Read the model definition and answer for the solid it produces. Units are mm, in the model's axes. A direction names the side the tool comes from. Coordinates: 2 decimals unless noted, no trailing zeros. Order: outer loops, then holes, each group sorted by start corner. A loop starts at its lowest first (then second) coordinate and runs counter-clockwise, first axis right, second up. Notation, with made-up numbers: (21, 56) -> (64, 56) arc R24 ccw to (64, 71) -> close; hole circle Ø3 at (72.25, 21). An arc over 180 degrees is marked (long way). Use CSV: the item, a comma, the result in double quotes.
```python
from build123d import *

# Parameters (mm, degrees)
SKETCH1_W           = 94
SKETCH1_H           = 48
BOSS_EXTRUDE1_DEPTH = 10
CUT_EXTRUDE1_DEPTH  = 6
SKETCH3_W           = 2.75
SKETCH3_H           = 8.5
CUT_EXTRUDE2_DEPTH  = 10
SKETCH4_R           = 2.5
BOSS_EXTRUDE2_DEPTH = 1.7
SKETCH5_R           = 2.5
BOSS_EXTRUDE3_DEPTH = 1.7
SKETCH6_R           = 2.5
CUT_EXTRUDE3_DEPTH  = 10
SKETCH11_R          = 3.2
CUT_EXTRUDE4_DEPTH  = 1
CUT_EXTRUDE5_START  = -10
SKETCH12_R          = 2.5
CUT_EXTRUDE5_DEPTH  = 10
CUT_EXTRUDE6_START  = -1
SKETCH13_R          = 3.2
CUT_EXTRUDE6_DEPTH  = 1
SKETCH15_W          = 20.2
SKETCH15_H          = 6.1
CUT_EXTRUDE7_DEPTH  = 2.1
CUT_EXTRUDE9_DEPTH  = 12
SKETCH19_W          = 11.1
SKETCH19_H          = 4.1
CUT_EXTRUDE10_DEPTH = 7.9
CUT_EXTRUDE11_DEPTH = 4.1


with BuildPart() as part:
    # Sketch1 → Boss-Extrude1 (new body)
    with BuildSketch(Plane(origin=(0, 0, 0), x_dir=(1, 0, 0), z_dir=(0, 1, 0))):
        Rectangle(SKETCH1_W, SKETCH1_H)
    extrude(amount=BOSS_EXTRUDE1_DEPTH)

    # Sketch2 → Cut-Extrude1 (cut)
    with BuildSketch(Plane(origin=(0, 10, 0), x_dir=(1, 0, 0), z_dir=(0, 1, 0))):
        Polygon((-21.568604419, -3.5), (-5.068604419, -3.5), (-5.068604419, -20), (-21.568604419, -20), (-21.568604419, -16), (-27.068604419, -16), (-27.068604419, -7.5), (-21.568604419, -7.5), align=None)
        Polygon((-21.5, 19), (-5, 19), (-5, 2.5), (-21.5, 2.5), (-21.5, 6.5), (-27, 6.5), (-27, 15), (-21.5, 15), align=None)
        Polygon((5, 19), (5, 2.5), (21.5, 2.5), (21.5, 6.5), (27, 6.5), (27, 15), (21.5, 15), (21.5, 19), align=None)
        Polygon((4.976902144, -3.5), (4.976902144, -20), (21.476902144, -20), (21.476902144, -16), (26.976902144, -16), (26.976902144, -7.5), (21.476902144, -7.5), (21.476902144, -3.5), align=None)
    extrude(amount=-CUT_EXTRUDE1_DEPTH, mode=Mode.SUBTRACT)

    # Sketch3 → Cut-Extrude2 (cut)
    with BuildSketch(Plane(origin=(0, 10, 0), x_dir=(1, 0, 0), z_dir=(0, 1, 0))):
        with Locations((25.625, 10.75)):
            Rectangle(SKETCH3_W, SKETCH3_H)
        with Locations((25.601902144, -11.75)):
            Rectangle(SKETCH3_W, SKETCH3_H)
        with Locations((-25.625, 10.75)):
            Rectangle(SKETCH3_W, SKETCH3_H)
        with Locations((-25.693604419, -11.75)):
            Rectangle(SKETCH3_W, SKETCH3_H)
    extrude(amount=-CUT_EXTRUDE2_DEPTH, mode=Mode.SUBTRACT)

    # Sketch4 → Boss-Extrude2 (add)
    with BuildSketch(Plane(origin=(0, 4, 0), x_dir=(1, 0, 0), z_dir=(0, 1, 0))):
        with Locations(Location((9.226902144, -7.75, 0), (0, 0, 270))):
            Circle(SKETCH4_R)
        with Locations(Location((9.226902144, -15.75, 0), (0, 0, 270))):
            Circle(SKETCH4_R)
        with Locations(Location((-9.318604419, -7.75, 0), (0, 0, 90))):
            Circle(SKETCH4_R)
        with Locations(Location((-9.318604419, -15.75, 0), (0, 0, 90))):
            Circle(SKETCH4_R)
        with Locations(Location((-9.25, 14.75, 0), (0, 0, 90))):
            Circle(SKETCH4_R)
        with Locations(Location((-9.25, 6.75, 0), (0, 0, 90))):
            Circle(SKETCH4_R)
        with Locations(Location((9.25, 14.75, 0), (0, 0, 270))):
            Circle(SKETCH4_R)
        with Locations(Location((9.25, 6.75, 0), (0, 0, 270))):
            Circle(SKETCH4_R)
    extrude(amount=BOSS_EXTRUDE2_DEPTH)

    # Sketch5 → Boss-Extrude3 (add)
    with BuildSketch(Plane(origin=(0, 10, 0), x_dir=(1, 0, 0), z_dir=(0, 1, 0))):
        with Locations(Location((-43, 20, 0), (0, 0, 270))):
            Circle(SKETCH5_R)
        with Locations(Location((-43, 12, 0), (0, 0, 270))):
            Circle(SKETCH5_R)
        with Locations(Location((-35, 20, 0), (0, 0, 270))):
            Circle(SKETCH5_R)
        with Locations(Location((-35, 12, 0), (0, 0, 270))):
            Circle(SKETCH5_R)
        with Locations(Location((-35, 4, 0), (0, 0, 270))):
            Circle(SKETCH5_R)
        with Locations(Location((-35, -4, 0), (0, 0, 270))):
            Circle(SKETCH5_R)
        with Locations(Location((-35, -12, 0), (0, 0, 270))):
            Circle(SKETCH5_R)
        with Locations(Location((-35, -20, 0), (0, 0, 270))):
            Circle(SKETCH5_R)
        with Locations(Location((-43, 4, 0), (0, 0, 270))):
            Circle(SKETCH5_R)
        with Locations(Location((-43, -4, 0), (0, 0, 270))):
            Circle(SKETCH5_R)
        with Locations(Location((-43, -12, 0), (0, 0, 270))):
            Circle(SKETCH5_R)
        with Locations(Location((-43, -20, 0), (0, 0, 270))):
            Circle(SKETCH5_R)
        with Locations(Location((43, -20, 0), (0, 0, 90))):
            Circle(SKETCH5_R)
        with Locations(Location((43, -12, 0), (0, 0, 90))):
            Circle(SKETCH5_R)
        with Locations(Location((43, -4, 0), (0, 0, 90))):
            Circle(SKETCH5_R)
        with Locations(Location((43, 4, 0), (0, 0, 90))):
            Circle(SKETCH5_R)
        with Locations(Location((35, -20, 0), (0, 0, 90))):
            Circle(SKETCH5_R)
        with Locations(Location((35, -12, 0), (0, 0, 90))):
            Circle(SKETCH5_R)
        with Locations(Location((35, -4, 0), (0, 0, 90))):
            Circle(SKETCH5_R)
        with Locations(Location((35, 4, 0), (0, 0, 90))):
            Circle(SKETCH5_R)
        with Locations(Location((35, 12, 0), (0, 0, 90))):
            Circle(SKETCH5_R)
        with Locations(Location((35, 20, 0), (0, 0, 90))):
            Circle(SKETCH5_R)
        with Locations(Location((43, 12, 0), (0, 0, 90))):
            Circle(SKETCH5_R)
        with Locations(Location((43, 20, 0), (0, 0, 90))):
            Circle(SKETCH5_R)
    extrude(amount=BOSS_EXTRUDE3_DEPTH)

    # Sketch6 → Cut-Extrude3 (cut)
    with BuildSketch(Plane.XY.offset(24)):
        with Locations((-43, 5)):
            Circle(SKETCH6_R)
        with Locations((-35, 5)):
            Circle(SKETCH6_R)
        with Locations(Location((35, 5, 0), (0, 0, 180))):
            Circle(SKETCH6_R)
        with Locations(Location((43, 5, 0), (0, 0, 180))):
            Circle(SKETCH6_R)
    extrude(amount=-CUT_EXTRUDE3_DEPTH, mode=Mode.SUBTRACT)

    # Sketch11 → Cut-Extrude4 (cut)
    with BuildSketch(Plane.XY.offset(24)):
        with Locations((-43, 5)):
            Circle(SKETCH11_R)
        with Locations((-35, 5)):
            Circle(SKETCH11_R)
        with Locations(Location((35, 5, 0), (0, 0, 180))):
            Circle(SKETCH11_R)
        with Locations(Location((43, 5, 0), (0, 0, 180))):
            Circle(SKETCH11_R)
    extrude(amount=-CUT_EXTRUDE4_DEPTH, mode=Mode.SUBTRACT)

    # Sketch12 → Cut-Extrude5 (cut)
    with BuildSketch(Plane(origin=(0, 0, -24), x_dir=(-1, 0, 0), z_dir=(0, 0, -1)).offset(CUT_EXTRUDE5_START)):
        with Locations((-43, 5)):
            Circle(SKETCH12_R)
        with Locations((-35, 5)):
            Circle(SKETCH12_R)
        with Locations(Location((35, 5, 0), (0, 0, 180))):
            Circle(SKETCH12_R)
        with Locations(Location((43, 5, 0), (0, 0, 180))):
            Circle(SKETCH12_R)
    extrude(amount=CUT_EXTRUDE5_DEPTH, mode=Mode.SUBTRACT)

    # Sketch13 → Cut-Extrude6 (cut)
    with BuildSketch(Plane(origin=(0, 0, -24), x_dir=(-1, 0, 0), z_dir=(0, 0, -1)).offset(CUT_EXTRUDE6_START)):
        with Locations((-43, 5)):
            Circle(SKETCH13_R)
        with Locations((-35, 5)):
            Circle(SKETCH13_R)
        with Locations(Location((35, 5, 0), (0, 0, 180))):
            Circle(SKETCH13_R)
        with Locations(Location((43, 5, 0), (0, 0, 180))):
            Circle(SKETCH13_R)
    extrude(amount=CUT_EXTRUDE6_DEPTH, mode=Mode.SUBTRACT)

    # Sketch15 → Cut-Extrude7 (cut)
    with BuildSketch(Plane(origin=(47, 0, 0), x_dir=(0, 0, -1), z_dir=(1, 0, 0))):
        with Locations((0, 3.05)):
            Rectangle(SKETCH15_W, SKETCH15_H)
    extrude(amount=-CUT_EXTRUDE7_DEPTH, mode=Mode.SUBTRACT)

    # Sketch17 → Cut-Extrude9 (cut)
    with BuildSketch(Plane.ZY.offset(47)):
        Polygon((-9.499804172, 0), (-12, 4.1), (-0.9, 4.1), (-3.399804172, 0), align=None)
        Polygon((0.9, 4.1), (3.399804172, 0), (9.499804172, 0), (12, 4.1), align=None)
    extrude(amount=-CUT_EXTRUDE9_DEPTH, mode=Mode.SUBTRACT)

    # Sketch19 → Cut-Extrude10 (cut)
    with BuildSketch(Plane.ZY.offset(35)):
        with Locations((-6.45, 2.05)):
            Rectangle(SKETCH19_W, SKETCH19_H)
        with Locations((6.45, 2.05)):
            Rectangle(SKETCH19_W, SKETCH19_H)
    extrude(amount=CUT_EXTRUDE10_DEPTH, mode=Mode.SUBTRACT)

    # Sketch16 → Cut-Extrude11 (cut)
    with BuildSketch(Plane(origin=(44.9, 0, 0), x_dir=(0, 0, -1), z_dir=(1, 0, 0))):
        Polygon((-5.8, 0), (-8.05, 4.1), (8.05, 4.1), (5.8, 0), align=None)
    extrude(amount=-CUT_EXTRUDE11_DEPTH, mode=Mode.SUBTRACT)


solid = part.part
```
Item 1: Find section C-C, the plane z = 0. Give the vertices of the cut face in (x, y), then the cut area to 3 significant figures.
Return value:
outline,"(-47, 0) -> (40.8, 0) -> (40.8, 4.1) -> (44.9, 4.1) -> (44.9, 6.1) -> (47, 6.1) -> (47, 10) -> (-47, 10) -> close"
area,"910 mm^2"
Item 2: Straight lines are drawn through the part: line 1 along X through (y, z) = (1.75, -8.5); line 2 along X through (y, z) = (7.5, 9); line 3 along Z through (x, y) = (-25, 4.5). For each, find the intervals that lie inside material, in ascending order.
Return value:
line 1,"x = -35 to -27, -24.25 to 24.25, 27 to 44.9"
line 2,"x = -47 to -27.07, -5.07 to 4.98, 26.98 to 47"
line 3,"z = -24 to -15, -6.5 to 7.5, 16 to 24"
Item 3: Find section B-B, the plane x = 18.5. Give the vertices of the cut face in (y, z), then the cut area to 3 significant figures.
Return value:
outline,"(0, -24) -> (10, -24) -> (10, -19) -> (4, -19) -> (4, -2.5) -> (10, -2.5) -> (10, 3.5) -> (4, 3.5) -> (4, 20) -> (10, 20) -> (10, 24) -> (0, 24) -> close"
area,"282 mm^2"
Item 4: A tool of negligible diameter and unlimited length cuts with its end or side. For faces 4 (the flat face through (42.88, 2.08, -6.94)), 5 (the cylindrical face through (-45.44, 10.84, 3.46)), 6 (the flat face through (-44.98, 2.08, 2.13)), from which of +Z, -Z, +X, -X, +Y, -Y can it reach the whole face along a straight path? Write none if from no direction.
Return value:
face 4,"+X"
face 5,"+Y"
face 6,"-X"
Item 5: Each of these flat-tipped pins is pushed along its axis until it touches: P1, Ø2, axis at y = 1.5, z = -2.5, coming from the +X side; P2, Ø6, axis at x = 22.5, z = 3, coming from the +Y side; P3, Ø5, axis at x = 43, y = 3.5, coming from the +Z side; P4, Ø1.5, axis at x = 7, z = -4.5, coming from the +Y side. Where does it stop, or does it pass through?
Return value:
P1,"stops at x = 40.8"
P2,"stops at y = 10"
P3,"stops at z = 24"
P4,"stops at y = 5.7"
Item 6: Find section D-D, the plane x = 0.5. Give the vertices of the cut face in (y, z), then the cut area to 3 significant figures.
Return value:
outline,"(0, -24) -> (10, -24) -> (10, 24) -> (0, 24) -> close"
area,"480 mm^2"
Item 7: Find section A-A, the plane z = -20. Give the vertices of the cut face in (x, y), then the cut area to 3 significant figures.
Return value:
outline,"(-47, 0) -> (47, 0) -> (47, 10) -> (45.5, 10) -> (45.5, 11.7) -> (40.5, 11.7) -> (40.5, 10) -> (37.5, 10) -> (37.5, 11.7) -> (32.5, 11.7) -> (32.5, 10) -> (-32.5, 10) -> (-32.5, 11.7) -> (-37.5, 11.7) -> (-37.5, 10) -> (-40.5, 10) -> (-40.5, 11.7) -> (-45.5, 11.7) -> (-45.5, 10) -> (-47, 10) -> close; hole circle Ø5 at (-43, 5); hole circle Ø5 at (-35, 5); hole circle Ø5 at (35, 5); hole circle Ø5 at (43, 5)"
area,"895 mm^2"
Item 8: The mould has two halves that part along Z. Classify faces 1 (the cylindrical face through (-40.69, 5.96, -18.44)), 2 (the flat face through (-35, 5, 14)), 3 (the flat face through (13, 7, -19)): +Z half, -Z half, draft (parallel to the pull), parting line (faces both ways), or undercut.
Return value:
face 1,"draft"
face 2,"+Z half"
face 3,"undercut"
